Work out the finished part from the listing and answer in its coordinate system (mm). A direction names the side the tool comes from. Give positions to 0.01 mm unless a question says otherwise; leave off trailing zeros. Loops run counter-clockwise (first coordinate to the right, second up) from the corner with the lowest first, then second, coordinate; pieces in that order, holes last. Notation, with made-up numbers: (14.25, -35) - (43.25, -35) arc R7 cw to (43.25, -23) - close; hole circle Ø8 at (56.25, -17.75). An arc over 180 degrees is marked (long way). One line per question, with ' | ' between items.
from build123d import *

# Parameters (mm, degrees)
SKETCH1_W           = 56.4
SKETCH1_H           = 56.4
SKETCH1_R           = 2.5
BOSS_EXTRUDE1_DEPTH = 5
BOSS_EXTRUDE2_DEPTH = 51
SKETCH3_R           = 5
CUT_EXTRUDE1_DEPTH  = 3
SKETCH5_R           = 3.175
BOSS_EXTRUDE3_DEPTH = 14
SKETCH6_R           = 19
BOSS_EXTRUDE4_DEPTH = 1.5
SKETCH7_R           = 5
CUT_EXTRUDE2_DEPTH  = 3
SKETCH9_R           = 3.175
BOSS_EXTRUDE5_DEPTH = 23
FILLET1_R           = 2
FILLET2_R           = 2
FILLET3_R           = 2
FILLET4_R           = 2
FILLET5_R           = 2
FILLET6_R           = 2
FILLET7_R           = 2
FILLET8_R           = 2
FILLET9_R           = 2
FILLET10_R          = 2
FILLET11_R          = 2
FILLET12_R          = 2
FILLET13_R          = 2
FILLET14_R          = 2
FILLET15_R          = 2
FILLET16_R          = 2


with BuildPart() as part:
    # Sketch1 → Boss-Extrude1 (new body)
    with BuildSketch(Plane(origin=(0, 0, 0), x_dir=(0, 0, -1), z_dir=(1, 0, 0))):
        Rectangle(SKETCH1_W, SKETCH1_H)
        with Locations((-23.57, 23.57)):
            Circle(SKETCH1_R, mode=Mode.SUBTRACT)
        with Locations((23.57, 23.57)):
            Circle(SKETCH1_R, mode=Mode.SUBTRACT)
        with Locations((23.57, -23.57)):
            Circle(SKETCH1_R, mode=Mode.SUBTRACT)
        with Locations((-23.57, -23.57)):
            Circle(SKETCH1_R, mode=Mode.SUBTRACT)
    extrude(amount=BOSS_EXTRUDE1_DEPTH)

    # Sketch2 → Boss-Extrude2 (add)
    with BuildSketch(Plane(origin=(5, 0, 0), x_dir=(0, 0, -1), z_dir=(1, 0, 0))):
        Polygon((-28.2, 19.2), (-19.2, 19.2), (-19.2, 28.2), (19.2, 28.2), (19.2, 19.2), (28.2, 19.2), (28.2, -19.2), (17.566571472, -19.2), (17.566571472, -28.2), (-19.2, -28.2), (-19.2, -19.2), (-28.2, -19.2), align=None)
    extrude(amount=BOSS_EXTRUDE2_DEPTH)

    # Sketch3 → Cut-Extrude1 (cut)
    with BuildSketch(Plane(origin=(56, 0, 0), x_dir=(0, 0, -1), z_dir=(1, 0, 0))):
        Circle(SKETCH3_R)
    extrude(amount=-CUT_EXTRUDE1_DEPTH, mode=Mode.SUBTRACT)

    # Sketch5 → Boss-Extrude3 (add)
    with BuildSketch(Plane(origin=(53, 0, 0), x_dir=(0, 0, -1), z_dir=(1, 0, 0))):
        Circle(SKETCH5_R)
    extrude(amount=BOSS_EXTRUDE3_DEPTH)

    # Sketch6 → Boss-Extrude4 (add)
    with BuildSketch(Plane.ZY):
        Circle(SKETCH6_R)
    extrude(amount=BOSS_EXTRUDE4_DEPTH)

    # Sketch7 → Cut-Extrude2 (cut)
    with BuildSketch(Plane.ZY.offset(1.5)):
        Circle(SKETCH7_R)
    extrude(amount=-CUT_EXTRUDE2_DEPTH, mode=Mode.SUBTRACT)

    # Sketch9 → Boss-Extrude5 (add)
    with BuildSketch(Plane.ZY.offset(-1.5)):
        Circle(SKETCH9_R)
    extrude(amount=BOSS_EXTRUDE5_DEPTH)

    # Fillet1
    fillet1_edges = [part.edges().sort_by_distance(p)[0] for p in [
        (2.5, 28.2, 28.2),
    ]]
    fillet(fillet1_edges, radius=FILLET1_R)

    # Fillet2
    fillet2_edges = [part.edges().sort_by_distance(p)[0] for p in [
        (2.5, 28.2, -28.2),
    ]]
    fillet(fillet2_edges, radius=FILLET2_R)

    # Fillet3
    fillet3_edges = [part.edges().sort_by_distance(p)[0] for p in [
        (2.5, -28.2, -28.2),
    ]]
    fillet(fillet3_edges, radius=FILLET3_R)

    # Fillet4
    fillet4_edges = [part.edges().sort_by_distance(p)[0] for p in [
        (2.5, -28.2, 28.2),
    ]]
    fillet(fillet4_edges, radius=FILLET4_R)

    # Fillet5
    fillet5_edges = [part.edges().sort_by_distance(p)[0] for p in [
        (30.5, 28.2, -19.2),
    ]]
    fillet(fillet5_edges, radius=FILLET5_R)

    # Fillet6
    fillet6_edges = [part.edges().sort_by_distance(p)[0] for p in [
        (30.5, 19.2, -28.2),
    ]]
    fillet(fillet6_edges, radius=FILLET6_R)

    # Fillet7
    fillet7_edges = [part.edges().sort_by_distance(p)[0] for p in [
        (30.5, -19.2, -28.2),
    ]]
    fillet(fillet7_edges, radius=FILLET7_R)

    # Fillet8
    fillet8_edges = [part.edges().sort_by_distance(p)[0] for p in [
        (30.5, -28.2, -17.566571472),
    ]]
    fillet(fillet8_edges, radius=FILLET8_R)

    # Fillet9
    fillet9_edges = [part.edges().sort_by_distance(p)[0] for p in [
        (30.5, -28.2, 19.2),
    ]]
    fillet(fillet9_edges, radius=FILLET9_R)

    # Fillet10
    fillet10_edges = [part.edges().sort_by_distance(p)[0] for p in [
        (30.5, -19.2, 28.2),
    ]]
    fillet(fillet10_edges, radius=FILLET10_R)

    # Fillet11
    fillet11_edges = [part.edges().sort_by_distance(p)[0] for p in [
        (30.5, 19.2, 28.2),
    ]]
    fillet(fillet11_edges, radius=FILLET11_R)

    # Fillet12
    fillet12_edges = [part.edges().sort_by_distance(p)[0] for p in [
        (30.5, 28.2, 19.2),
    ]]
    fillet(fillet12_edges, radius=FILLET12_R)

    # Fillet13
    fillet13_edges = [part.edges().sort_by_distance(p)[0] for p in [
        (30.5, 19.2, -19.2),
    ]]
    fillet(fillet13_edges, radius=FILLET13_R)

    # Fillet14
    fillet14_edges = [part.edges().sort_by_distance(p)[0] for p in [
        (30.5, -19.2, -17.566571472),
    ]]
    fillet(fillet14_edges, radius=FILLET14_R)

    # Fillet15
    fillet15_edges = [part.edges().sort_by_distance(p)[0] for p in [
        (30.5, -19.2, 19.2),
    ]]
    fillet(fillet15_edges, radius=FILLET15_R)

    # Fillet16
    fillet16_edges = [part.edges().sort_by_distance(p)[0] for p in [
        (30.5, 19.2, 19.2),
    ]]
    fillet(fillet16_edges, radius=FILLET16_R)


solid = part.part
1. Find section C-C on x = 28. Write down the section's boundary in (y, z), then the cut area to 3 significant figures.
Evaluation:
outline: (-28.2, -15.57) arc R2 ccw to (-26.2, -17.57) - (-21.2, -17.57) arc R2 cw to (-19.2, -19.57) - (-19.2, -26.2) arc R2 ccw to (-17.2, -28.2) - (17.2, -28.2) arc R2 ccw to (19.2, -26.2) - (19.2, -21.2) arc R2 cw to (21.2, -19.2) - (26.2, -19.2) arc R2 ccw to (28.2, -17.2) - (28.2, 17.2) arc R2 ccw to (26.2, 19.2) - (21.2, 19.2) arc R2 cw to (19.2, 21.2) - (19.2, 26.2) arc R2 ccw to (17.2, 28.2) - (-17.2, 28.2) arc R2 ccw to (-19.2, 26.2) - (-19.2, 21.2) arc R2 cw to (-21.2, 19.2) - (-26.2, 19.2) arc R2 ccw to (-28.2, 17.2) - close | area: 2,840 mm2
2. Flat-ended cylindrical pins translate along their axes: pin 1 (5.5 mm diameter, centred on x = 37, y = -24, fed in from -Z); pin 2 (4 mm diameter, centred on x = 22, y = 24, fed in from -Z); pin 3 (9 mm diameter, centred on y = -21.5, z = -21, fed in from +X). Find the tip coordinate at first contact, or state that the pin passes through.
Evaluation:
pin 1: z = -17.57 | pin 2: z = -19.2 | pin 3: x = 56
3. Find section A-A on z = -23.57. Write down the section's boundary in (x, y).
Evaluation:
outline: (0, -28.2) - (5, -28.2) - (5, -26.07) - (0, -26.07) - close; (0, -21.07) - (5, -21.07) - (5, -19.2) - (56, -19.2) - (56, 19.2) - (5, 19.2) - (5, 21.07) - (0, 21.07) - close; (0, 26.07) - (5, 26.07) - (5, 28.2) - (0, 28.2) - close
4. Find section B-B on y = -23.57. Write down the section's boundary in (x, z).
Evaluation:
outline: (0, -28.2) - (5, -28.2) - (5, -26.07) - (0, -26.07) - close; (0, -21.07) - (5, -21.07) - (5, -17.57) - (56, -17.57) - (56, 19.2) - (5, 19.2) - (5, 21.07) - (0, 21.07) - close; (0, 26.07) - (5, 26.07) - (5, 28.2) - (0, 28.2) - close
5. Find section D-D on z = 0. Write down the section's boundary in (x, y) (3 decimals), then the cut area to 3 significant figures.
Evaluation:
outline: (-21.5, -3.175) - (1.5, -3.175) - (1.5, -5) - (-1.5, -5) - (-1.5, -19) - (0, -19) - (0, -28.2) - (56, -28.2) - (56, -5) - (53, -5) - (53, -3.175) - (67, -3.175) - (67, 3.175) - (53, 3.175) - (53, 5) - (56, 5) - (56, 28.2) - (0, 28.2) - (0, 19) - (-1.5, 19) - (-1.5, 5) - (1.5, 5) - (1.5, 3.175) - (-21.5, 3.175) - close | area: 3,390 mm2
6. Determine the mould class of faces 6 (the cylindrical face through (2.465, -25.091, -21.586)), 7 (the cylindrical face through (30.86, 19.77, 19.8)), 8 (the flat face through (67, 0, 0)) for opening direction Y: +Y half, -Y half, draft (parallel to the pull), parting line (faces both ways), or undercut.
Evaluation:
face 6: undercut | face 7: +Y half | face 8: draft
7. Consider L1, parallel to Y at x = 2.2, z = 23.57; L2, parallel to Y at x = 55.05, z = 0 (3 decimals); L3, parallel to Z at x = 3, y = 23. Determine where each line is inside the solid, lowest interval first.
Evaluation:
L1: -28.2 to -26.07, -21.07 to 21.07, 26.07 to 28.2 | L2: -28.2 to -5, -3.175 to 3.175, 5 to 28.2 | L3: -28.2 to -26, -21.14 to 21.14, 26 to 28.2
8. Which of the six approach directions +Z, -Z, +X, -X, +Y, -Y give full straight-line access (tool end or side, diameter ignored) to faces 1 (the flat face through (5, -24, -20)), 2 (the flat face through (30, 19.2, -24)), 3 (the cylindrical face through (30.86, -18.6, 27.63)), 4 (the flat face through (5, 24, 26.4)), 5 (the cylindrical face through (-0.74, -16.856, 8.767))?
Evaluation:
face 1: -Z, +X, -Y | face 2: -Z, +X, +Y | face 3: +Z, +X, -Y | face 4: +Z, +X, +Y | face 5: -X
